Input: part model. Units: mm. Frame: model coordinates. A direction names the side the tool comes from. Coordinates: 2 decimals unless noted, no trailing zeros. Order: outer loops, then holes, each group sorted by start corner. A loop starts at its lowest first (then second) coordinate and runs counter-clockwise, first axis right, second up.
from build123d import *

# Parameters (mm, degrees)
BOSS_EXTRUDE1_DEPTH = 75
SKETCH3_W           = 10
SKETCH3_H           = 10
CUT_EXTRUDE1_DEPTH  = 10
SKETCH4_R           = 2
CUT_EXTRUDE2_DEPTH  = 11
CHAMFER1_SIZE       = 1.5
CHAMFER2_SIZE       = 1


with BuildPart() as part:
    # Sketch2 → Boss-Extrude1 (new body)
    with BuildSketch(Plane.XY):
        Polygon((13, 50), (13, 10), (21, 10), (21, 0), (0, 0), (0, 50), align=None)
    extrude(amount=BOSS_EXTRUDE1_DEPTH)

    # Sketch3 → Cut-Extrude1 (cut)
    with BuildSketch(Plane(origin=(0, 50, 0), x_dir=(1, 0, 0), z_dir=(0, 1, 0))):
        with Locations((6.5, -6.5)):
            Rectangle(SKETCH3_W, SKETCH3_H)
        with Locations((6.5, -68.5)):
            Rectangle(SKETCH3_W, SKETCH3_H)
    extrude(amount=-CUT_EXTRUDE1_DEPTH, mode=Mode.SUBTRACT)

    # Sketch4 → Cut-Extrude2 (cut, through all)
    with BuildSketch(Plane(origin=(0, 10, 0), x_dir=(1, 0, 0), z_dir=(0, 1, 0))):
        with Locations((17, -5.5)):
            Circle(SKETCH4_R)
        with Locations((17, -37.5)):
            Circle(SKETCH4_R)
        with Locations((17, -69.5)):
            Circle(SKETCH4_R)
    extrude(amount=-CUT_EXTRUDE2_DEPTH, mode=Mode.SUBTRACT)

    # Chamfer1
    chamfer1_edges = [part.edges().sort_by_distance(p)[0] for p in [
        (21, 5, 75),
        (21, 5, 0),
    ]]
    chamfer(chamfer1_edges, length=CHAMFER1_SIZE)

    # Chamfer2
    chamfer2_edges = [part.edges().sort_by_distance(p)[0] for p in [
        (0, 25, 75),
        (0, 25, 0),
    ]]
    chamfer(chamfer2_edges, length=CHAMFER2_SIZE)


solid = part.part
Item 1: Cut plane D-D on x = 8.25. Return loops of the section in (y, z).
Response values:
outline: (0, 0) - (50, 0) - (50, 1.5) - (40, 1.5) - (40, 11.5) - (50, 11.5) - (50, 63.5) - (40, 63.5) - (40, 73.5) - (50, 73.5) - (50, 75) - (0, 75) - close
Item 2: Pin query (flat end, axial travel): pin 1 Ø4 at (x, z) = (15.5, 60) entering from -Y; pin 2 Ø4 at (y, z) = (35.5, 16) entering from +X; pin 3 Ø4 at (x, y) = (15.5, 28) entering from -Z; pin 4 Ø5 at (x, z) = (5, 69.5) entering from +Y. Return the tip coordinate at first contact, or that it passes through.
Response values:
pin 1: stops at y = 0
pin 2: stops at x = 13
pin 3: passes through
pin 4: stops at y = 40
Item 3: Access query for faces 4 (the face through (8, 25, 0)), 5 (the face through (13, 30, 37)), 6 (the face through (11.5, 45, 69)). Directions: +Z, -Z, +X, -X, +Y, -Y. A direction counts if a zero-diameter tool reaches every point of the face in a straight line with its end or side. Return the directions, or none.
Response values:
face 4: -Z, +X, -X, +Y, -Y
face 5: +Z, -Z, +X, +Y
face 6: +Y
Item 4: Ray query, probe 1 along Z at (x, y) = (17, 2); probe 2 along Z at (x, y) = (7.25, 46.5); probe 3 along Y at (x, z) = (19.25, 69.5). Return the intervals inside material, ascending.
Response values:
probe 1: z = 0 to 3.5, 7.5 to 35.5, 39.5 to 67.5, 71.5 to 75
probe 2: z = 0 to 1.5, 11.5 to 63.5, 73.5 to 75
probe 3: y = 0 to 10
Item 5: Draft query along Z for faces 1 (the face through (14, 10, 37)), 2 (the face through (20.3, 5.1, 0.8)), 3 (the face through (1.5, 45, 69)). Return one class per face: pulls with the +Z half, pulls with the -Z half, needs draft (parallel to the pull), parting line crosses it, or undercut.
Response values:
face 1: needs draft
face 2: pulls with the -Z half
face 3: undercut
Item 6: Cut plane B-B on y = 3.5. Return loops of the section in (x, z), then the cut area to 3 significant figures.
Response values:
outline: (0, 1) - (1, 0) - (19.5, 0) - (21, 1.5) - (21, 73.5) - (19.5, 75) - (1, 75) - (0, 74) - close; hole circle Ø4 at (17, 5.5); hole circle Ø4 at (17, 37.5); hole circle Ø4 at (17, 69.5)
area: 1,530 mm2
Item 7: Cut plane C-C on x = 17. Return loops of the section in (y, z).
Response values:
outline: (0, 0) - (10, 0) - (10, 3.5) - (0, 3.5) - close; (0, 7.5) - (10, 7.5) - (10, 35.5) - (0, 35.5) - close; (0, 39.5) - (10, 39.5) - (10, 67.5) - (0, 67.5) - close; (0, 71.5) - (10, 71.5) - (10, 75) - (0, 75) - close
Item 8: Cut plane A-A on z = 37.5. Return loops of the section in (x, y).
Response values:
outline: (0, 0) - (15, 0) - (15, 10) - (13, 10) - (13, 50) - (0, 50) - close; (19, 0) - (21, 0) - (21, 10) - (19, 10) - close
